from build123d import *

# Parameters (mm, degrees)
SKETCH_1_W                     = 25
SKETCH_1_H                     = 25
SKETCH_1_W_2                   = 19
SKETCH_1_H_2                   = 19
EXTRUDE_1_DEPTH                = 1390
HOLE_WIZARD_6_0_6_1_AT_2_COUNT = 2
HOLE_WIZARD_6_0_6_1_AT_2_PITCH = 70
CUT_EXTRUDE_1_REACH            = 1392.45
SKETCH_6_R                     = 6
PATTERN_LINEAR_1_COUNT         = 2
PATTERN_LINEAR_1_PITCH         = 1296.34


with BuildPart() as part:
    # Sketch 1 → Extrude 1 (new body)
    with BuildSketch(Plane.XY):
        with Locations((12.5, -12.5)):
            Rectangle(SKETCH_1_W, SKETCH_1_H)
        with Locations((12.5, -12.5)):
            Rectangle(SKETCH_1_W_2, SKETCH_1_H_2, mode=Mode.SUBTRACT)
    extrude(amount=EXTRUDE_1_DEPTH)

    # Sketch 4 → Hole Wizard 6.0 _6_ _1 (revolve, cut)
    with BuildSketch(Plane(origin=(0, -12.5, 11.8), x_dir=(0, 0, 1), z_dir=(0, 1, 0))):
        Polygon((0, 0), (0, 31.802581857), (3, 30), (3, 0), align=None)
    hole_wizard_6_0_6_1 = revolve(axis=Axis((-6.35, -12.5, 11.8), (1, 0, 0)), mode=Mode.SUBTRACT)

    # Hole Wizard 6.0 _6_ _1 at 2: Hole Wizard 6.0 _6_ _1 ×2
    with Locations(*[(0, 0, i * HOLE_WIZARD_6_0_6_1_AT_2_PITCH) for i in range(1, HOLE_WIZARD_6_0_6_1_AT_2_COUNT)]):
        add(hole_wizard_6_0_6_1, mode=Mode.SUBTRACT)

    # Sketch 6 → Cut-Extrude 1 (cut, up to next)
    with BuildSketch(Plane(origin=(25, 0, 0), x_dir=(0, 0, -1), z_dir=(1, 0, 0)), mode=Mode.PRIVATE) as cut_extrude_1_sk1:
        with Locations(Location((-11.8, -12.5, 0), (0, 0, 90))):
            Circle(SKETCH_6_R)
    cut_extrude_1_tool1 = extrude(cut_extrude_1_sk1.sketch, amount=-CUT_EXTRUDE_1_REACH, mode=Mode.PRIVATE) & part.part
    # Sketch 6 → Cut-Extrude 1 (cut, up to next)
    with BuildSketch(Plane(origin=(25, 0, 0), x_dir=(0, 0, -1), z_dir=(1, 0, 0)), mode=Mode.PRIVATE) as cut_extrude_1_sk2:
        with Locations(Location((-81.8, -12.5, 0), (0, 0, 90))):
            Circle(SKETCH_6_R)
    cut_extrude_1_tool2 = extrude(cut_extrude_1_sk2.sketch, amount=-CUT_EXTRUDE_1_REACH, mode=Mode.PRIVATE) & part.part
    cut_extrude_1_1 = cut_extrude_1_tool1.solids().sort_by_distance((25, -12.5, 11.8))[0]
    add(cut_extrude_1_1, mode=Mode.SUBTRACT)
    cut_extrude_1_2 = cut_extrude_1_tool2.solids().sort_by_distance((25, -12.5, 81.8))[0]
    add(cut_extrude_1_2, mode=Mode.SUBTRACT)
    cut_extrude_1 = cut_extrude_1_1 + cut_extrude_1_2  # Cut-Extrude 1 as one shape, for the pattern or mirror that repeats it

    # Pattern Linear 1: Hole Wizard 6.0 _6_ _1, Cut-Extrude 1 ×2
    with Locations(*[(0, 0, i * PATTERN_LINEAR_1_PITCH) for i in range(1, PATTERN_LINEAR_1_COUNT)]):
        add(hole_wizard_6_0_6_1, mode=Mode.SUBTRACT)
        add(cut_extrude_1, mode=Mode.SUBTRACT)

    # Pattern Linear 1 copy 1 sketch → Pattern Linear 1 copy 1 (revolve, cut)
    with BuildSketch(Plane(origin=(0, -12.5, 1378.14), x_dir=(0, 0, 1), z_dir=(0, 1, 0))):
        Polygon((0, 0), (0, 31.802581857), (3, 30), (3, 0), align=None)
    revolve(axis=Axis((-6.35, -12.5, 1378.14), (1, 0, 0)), mode=Mode.SUBTRACT)


solid = part.part
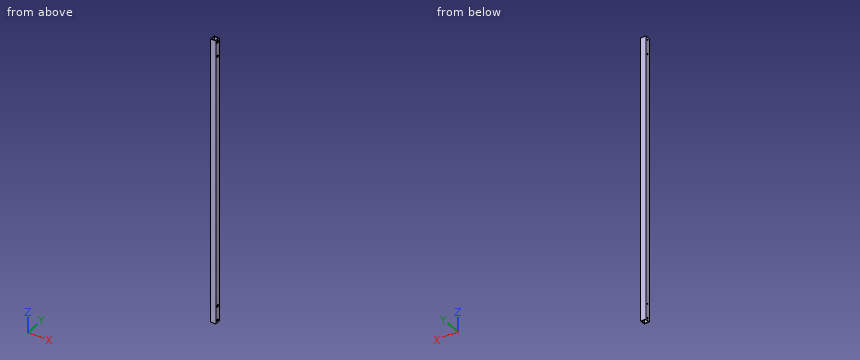
Part model, mm, in its own coordinate system. Round coordinates to 2 decimals unless told otherwise and drop trailing zeros. Order: outer loops, then holes, each group sorted by start corner. A loop starts at its lowest first (then second) coordinate and runs counter-clockwise, first axis right, second up. Notation, with made-up numbers: (-33, -17.75) -> (16, -17.75) arc R10 cw to (16, -4.75) -> close; hole circle Ø7 at (13, -8). An arc over 180 degrees is marked (long way). Put each result on its own line as item: value.
Q1. Wall check: line 1 (Z direction, x = 1.8, y = -12.5); line 2 (X direction, y = -21.5, z = 296.5); line 3 (Z direction, x = 23.7, y = -12.5). Give the ranges that are in metal, low to high. Write a range as [from, to].
From the geometry:
line 1: z = [0, 8.8], [14.8, 78.8], [84.8, 1305.14], [1311.14, 1375.14], [1381.14, 1390]
line 2: x = [0, 3], [22, 25]
line 3: z = [0, 5.8], [17.8, 75.8], [87.8, 1302.14], [1314.14, 1372.14], [1384.14, 1390]
Q2. Pin check, flat tip, straight feed: pin 1 Ø8 at (y, z) = (-12.5, 1378.14) entering from +X. Stop position of the tip, or through.
From the geometry:
pin 1: stops at x = 3
Q3. Band-saw the part on A-A (x = 12). Give the cut face in (y, z).
From the geometry:
outline: (-25, 0) -> (-22, 0) -> (-22, 1390) -> (-25, 1390) -> close; (-3, 0) -> (0, 0) -> (0, 1390) -> (-3, 1390) -> close
Q4. Band-saw the part on B-B (z = 273). Give the cut face in (x, y), and give its area (3 significant figures).
From the geometry:
outline: (0, -25) -> (25, -25) -> (25, 0) -> (0, 0) -> close; hole (3, -22) -> (22, -22) -> (22, -3) -> (3, -3) -> close
area: 264 mm2
